Here's the drawing with two shaded views (mm, measured from the low corner). I have some questions. A direction names the side the tool comes from. Round coordinates to 2 decimals unless told otherwise and drop trailing zeros. Write each loop counter-clockwise with the first axis right and the second up, starting at its lowest first coordinate (ties: lowest second). Pieces come first, ordered by that corner, then holes. Notation, with made-up numbers: M 5.5,57 L 49.5,57 A15 ccw 49.5,62 Z; hole C -37,78.25 d6. An arc over 180 degrees is marked long. Answer as a JSON object with one key per item and string values. Group by question number.
1) Suppose I cut it at A-A, the plane x = 203.2. Write out the boundary of the cut face in (y, z).
2) On a 3-axis mill with a long thin cutter (end or side, diameter ignored), from which of +Z, -Z, +X, -X, +Y, -Y can I reach the whole of each face in a straight line? I mean the marked faces 1, 2, 3, 4 and 5. Say none if no direction works.
3) Suppose I cut it at B-B, the plane y = 68. Write out the boundary of the cut face in (x, z).
4) Suppose I cut it at C-C, the plane x = 295.5. Write out the boundary of the cut face in (y, z).
5) Please list where these lines run through material, in increasing order: L1, parallel to Y at x = 252.5, z = 551; L2, parallel to Y at x = 292.5, z = 183; L3, parallel to Z at x = 208, y = 185. Write a range as [from, to].
6) If we mould it in two halves opening along Y, with no side actions, what happens to the marked faces 6, 7 and 8? For each: +Y half, -Y half, draft (parallel to the pull), parting line (faces both ways), or undercut.
7) I'm going to push flat-ended pins straight in: pin 1 Ø6 at (x, z) = (54.5, 575.5) entering from +Y; pin 2 Ø1.5 at (y, z) = (536, 529.5) entering from -X; pin 3 Ø3 at (x, y) = (197.5, 377.5) entering from +Z. Where does each tip first touch, or does it pass through?
8) Suppose I cut it at D-D, the plane z = 591. Write out the boundary of the cut face in (x, y) (3 decimals), and give its area (3 significant figures).
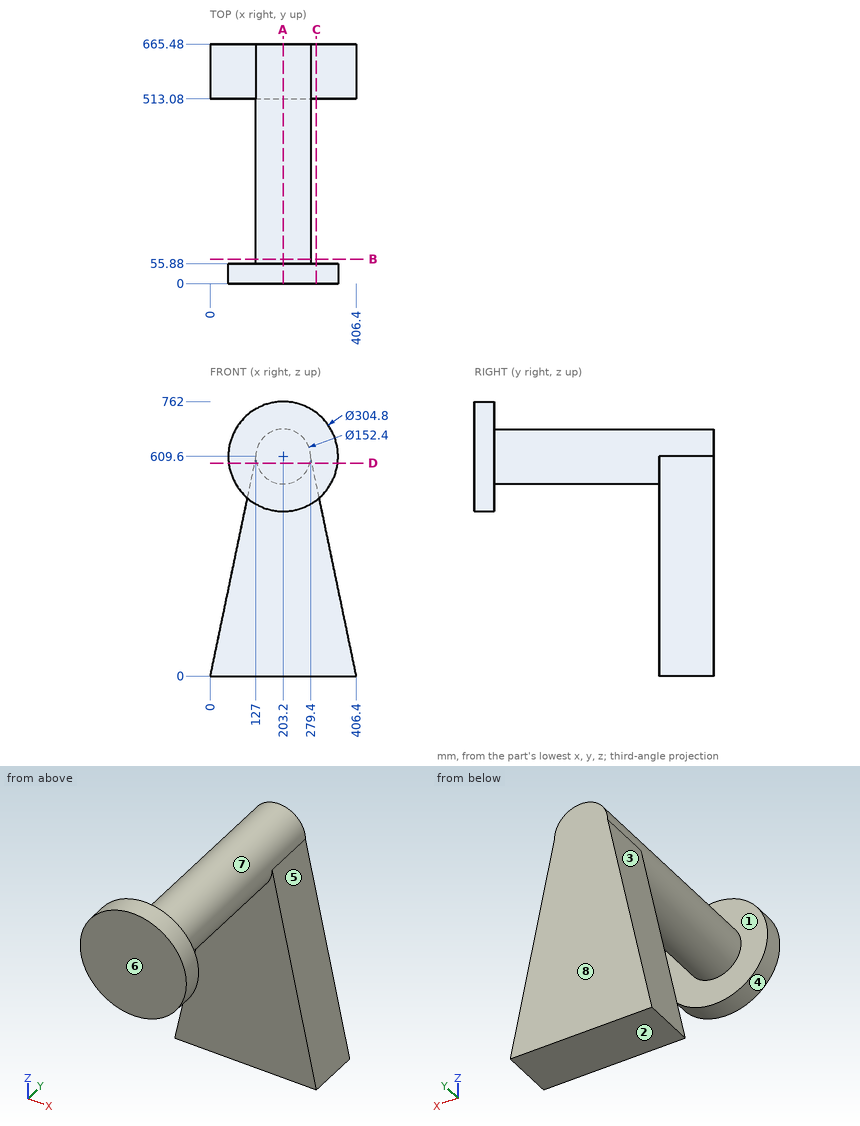
Results:
{
 "1": {"outline": "M 0,457.2 L 55.88,457.2 L 55.88,533.4 L 513.08,533.4 L 513.08,0 L 665.48,0 L 665.48,685.8 L 55.88,685.8 L 55.88,762 L 0,762 Z"},
 "2": {"face 1": "none", "face 2": "-Z, +X, -X, +Y, -Y", "face 3": "+Z, -X, +Y", "face 4": "-Y", "face 5": "+Z, +X, +Y"},
 "3": {"outline": "C 203.2,609.6 d152.4"},
 "4": {"outline": "M 0,488.33 L 55.88,488.33 L 55.88,730.87 L 0,730.87 Z; M 513.08,0 L 665.48,0 L 665.48,532.32 L 513.08,532.32 Z"},
 "5": {"L1": "[0, 55.88], [513.08, 665.48]", "L2": "[513.08, 665.48]", "L3": "[533.55, 685.65]"},
 "6": {"face 6": "-Y half", "face 7": "undercut", "face 8": "+Y half"},
 "7": {"pin 1": "y = 55.88", "pin 2": "x = 110.16", "pin 3": "z = 685.68"},
 "8": {"outline": "M 51.939,0 L 354.461,0 L 354.461,55.88 L 277.095,55.88 L 277.095,513.08 L 283.275,513.08 L 283.275,665.48 L 123.125,665.48 L 123.125,513.08 L 129.305,513.08 L 129.305,55.88 L 51.939,55.88 Z", "area": "109,000 mm^2"}
}
